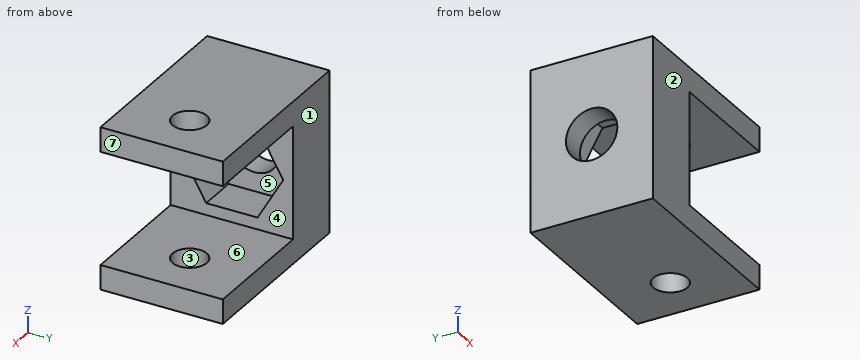
from build123d import *

# Parameters (mm, degrees)
BOSS_EXTRU_1_DEPTH      = 25
ESQUISSE3_R             = 3.5
ENL_V_MAT_EXTRU_1_DEPTH = 57.196085273
ESQUISSE4_R             = 5.25
ENL_V_MAT_EXTRU_2_DEPTH = 49.363209157
ENL_V_MAT_EXTRU_3_DEPTH = 8


with BuildPart() as part:
    # Esquisse2 → Boss.-Extru.1 (new body)
    with BuildSketch(Plane(origin=(0, 0, 0), x_dir=(1, 0, 0), z_dir=(0, 1, 0))):
        Polygon((0, 0), (-38, 0), (-38, -33), (0, -33), (0, -28), (-25, -28), (-25, -5), (0, -5), align=None)
    extrude(amount=BOSS_EXTRU_1_DEPTH)

    # Esquisse3 → Enlèv. mat.-Extru.1 (cut, through all)
    with BuildSketch(Plane.XY.offset(33)):
        with Locations((-10, 12.5)):
            Circle(ESQUISSE3_R)
    extrude(amount=-ENL_V_MAT_EXTRU_1_DEPTH, mode=Mode.SUBTRACT)

    # Esquisse4 → Enlèv. mat.-Extru.2 (cut, through all)
    with BuildSketch(Plane(origin=(-25, 0, 0), x_dir=(0, 0, -1), z_dir=(1, 0, 0))):
        with Locations((-16.5, 12.5)):
            Circle(ESQUISSE4_R)
    extrude(amount=-ENL_V_MAT_EXTRU_2_DEPTH, mode=Mode.SUBTRACT)

    # Esquisse5 → Enlèv. mat.-Extru.3 (cut)
    with BuildSketch(Plane(origin=(-25, 0, 0), x_dir=(0, 0, -1), z_dir=(1, 0, 0))):
        Polygon((-7.40673326, 17.75), (-16.5, 23), (-25.59326674, 17.75), (-25.59326674, 7.25), (-16.5, 2), (-7.40673326, 7.25), align=None)
    extrude(amount=-ENL_V_MAT_EXTRU_3_DEPTH, mode=Mode.SUBTRACT)


solid = part.part
Could you check a few things on this model? Use its own coordinates, in mm. Face numbers are marked on the shaded views. A direction names the side the tool comes from. Give positions to 0.01 mm unless a question says otherwise; leave off trailing zeros. Write each loop counter-clockwise with the first axis right and the second up, starting at its lowest first coordinate (ties: lowest second). Pieces come first, ordered by that corner, then holes. Notation, with made-up numbers: (60.25, 0) -> (109.25, 0) arc R13 cw to (109.25, 21) -> close; hole circle Ø9 at (63.25, 58). An arc over 180 degrees is marked (long way). Write each question's results on one line, items separated by ' | '. Start each with the question number.
Q1. I need wall thicknesses on probe 1 along Z at (x, y) = (-32, 16.5); probe 2 along Z at (x, y) = (-23, 18.25); probe 3 along Y at (x, z) = (-10, 31). Which ranges of each line are inside material? Lowest first, please.
Q2. Suppose I cut it at C-C, the plane z = 28.5. List the corners of the cut face in (x, y) for me.
Q3. We'd pull the mould along Y, two halves only. Please class the marked faces 1, 2, 3 and 4: +Y half, -Y half, draft (parallel to the pull), parting line (faces both ways), or undercut.
Q4. Suppose I cut it at A-A, the plane y = 12.5. List the corners of the cut face in (x, z) for me.
Q5. I'm going to push flat-ended pins straight in: pin 1 Ø14.5 at (y, z) = (9, 16.5) entering from +X; pin 2 Ø6 at (x, z) = (-11.5, 24.5) entering from -Y. Where does each tip first touch, or does it pass through?
Q6. Suppose I cut it at B-B, the plane x = -10. List the corners of the cut face in (y, z) for me.
Q7. Suppose I cut it at D-D, the plane x = -26.5. List the corners of the cut face in (y, z) for me, and give its area (3 significant figures).
Q8. Which directions (+Z, -Z, +X, -X, +Y, -Y) give clear straight access to the entire face, cutting with the end or side of a thin tool? Please do the marked faces 5, 6 and 7.
Outcome:
1) probe 1: 0 to 7.41, 25.59 to 33 | probe 2: 0 to 5, 28 to 33 | probe 3: 0 to 9, 16 to 25
2) outline: (-38, 0) -> (0, 0) -> (0, 25) -> (-38, 25) -> close; hole circle Ø7 at (-10, 12.5)
3) face 1: +Y half | face 2: -Y half | face 3: undercut | face 4: draft
4) outline: (-38, 0) -> (-13.5, 0) -> (-13.5, 5) -> (-25, 5) -> (-25, 7.41) -> (-33, 7.41) -> (-33, 11.25) -> (-38, 11.25) -> close; (-38, 21.75) -> (-33, 21.75) -> (-33, 25.59) -> (-25, 25.59) -> (-25, 28) -> (-13.5, 28) -> (-13.5, 33) -> (-38, 33) -> close; (-6.5, 0) -> (0, 0) -> (0, 5) -> (-6.5, 5) -> close; (-6.5, 28) -> (0, 28) -> (0, 33) -> (-6.5, 33) -> close
5) pin 1: x = -25 | pin 2: through
6) outline: (0, 0) -> (9, 0) -> (9, 5) -> (0, 5) -> close; (0, 28) -> (9, 28) -> (9, 33) -> (0, 33) -> close; (16, 0) -> (25, 0) -> (25, 5) -> (16, 5) -> close; (16, 28) -> (25, 28) -> (25, 33) -> (16, 33) -> close
7) outline: (0, 0) -> (25, 0) -> (25, 33) -> (0, 33) -> close; hole (2, 16.5) -> (7.25, 7.41) -> (17.75, 7.41) -> (23, 16.5) -> (17.75, 25.59) -> (7.25, 25.59) -> close | area: 539 mm2
8) face 5: +X | face 6: +X, +Y, -Y | face 7: +Z, -Z, +X, +Y, -Y
